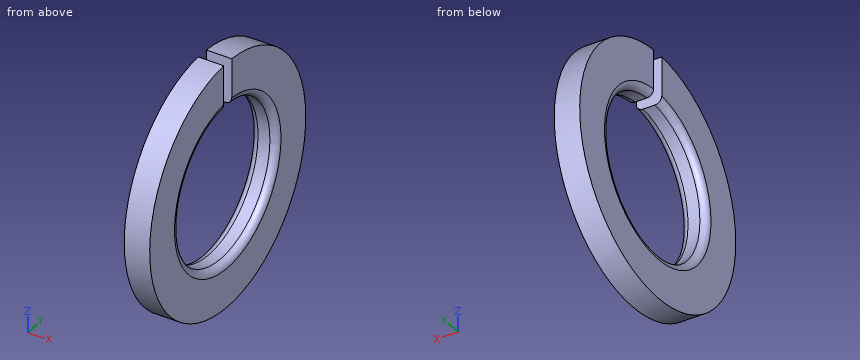
from build123d import *

# Parameters (mm, degrees)
SKETCH2_W = 3
SKETCH2_H = 29.682
GAP_DEPTH = 42.588700388


with BuildPart() as part:
    # Sketch1 → Base-Revolve (revolve)
    with BuildSketch(Plane.XY, mode=Mode.PRIVATE) as base_revolve_sk:
        with BuildLine():
            Line((0, 19.85), (0, 29.1))
            Line((0, 29.1), (-6, 29.1))
            Line((-6, 29.1), (-6, 19.85))
            ThreePointArc((-6, 19.85), (-5.53137085, 18.71862915), (-4.4, 18.25))
            Line((-4.4, 18.25), (-1.6, 18.25))
            ThreePointArc((-1.6, 18.25), (-0.46862915, 18.71862915), (0, 19.85))
        make_face()
    revolve(base_revolve_sk.sketch.rotate(Axis((-34.925, 0, 0), (1, 0, 0)), 90), axis=Axis((-34.925, 0, 0), (1, 0, 0)))

    # Sketch2 → Gap (cut, through all)
    with BuildSketch(Plane(origin=(0, 0, 0), x_dir=(0, -1, 0), z_dir=(-1, 0, 0))):
        with Locations((0, 14.841)):
            Rectangle(SKETCH2_W, SKETCH2_H)
    extrude(amount=GAP_DEPTH, mode=Mode.SUBTRACT)


solid = part.part
Here's how the part is built. I have some questions about the finished solid (model axes, mm). Round coordinates to 2 decimals unless told otherwise and drop trailing zeros. Loops run counter-clockwise (first coordinate to the right, second up) from the corner with the lowest first, then second, coordinate; pieces in that order, holes last. Notation, with made-up numbers: (83.25, -15.75) - (139.25, -15.75) arc R18 ccw to (139.25, 13.25) - close; hole circle Ø7 at (62.5, -20.5). An arc over 180 degrees is marked (long way). One line per question, with ' | ' between items. Start each with the question number.
Q1. I want a section at A-A (z = 0). Write out the boundary of the cut face in (x, y).
Q2. I want a section at B-B (y = 0). Write out the boundary of the cut face in (x, z).
Q3. Please list where these lines run through material, in increasing order: line 1 (Y direction, x = -2.25, z = 0); line 2 (Z direction, x = -2.5, y = -10); line 3 (Z direction, x = -3.75, y = -8.5). Write a range as [from, to].
Q4. I want a section at C-C (x = -3.5). Write out the boundary of the cut face in (y, z), then the cut area to 3 significant figures.
Q5. I want a section at D-D (z = 24). Write out the boundary of the cut face in (x, y), then the cut area to 3 significant figures.
Q6. Will these pins go through, and if not, where does the flat tip stop? pin 1 (1.5 mm diameter, centred on x = -3, z = -12, fed in from -Y); pin 2 (2 mm diameter, centred on x = -3.5, z = 23, fed in from -Y); pin 3 (1.8 mm diameter, centred on x = -3, z = 25.5, fed in from +Y).
Response values:
1) outline: (-6, -29.1) - (0, -29.1) - (0, -19.85) arc R1.6 ccw to (-1.6, -18.25) - (-4.4, -18.25) arc R1.6 ccw to (-6, -19.85) - close; (-6, 19.85) arc R1.6 ccw to (-4.4, 18.25) - (-1.6, 18.25) arc R1.6 ccw to (0, 19.85) - (0, 29.1) - (-6, 29.1) - close
2) outline: (-6, -29.1) - (0, -29.1) - (0, -19.85) arc R1.6 ccw to (-1.6, -18.25) - (-4.4, -18.25) arc R1.6 ccw to (-6, -19.85) - close
3) line 1: y = [-29.1, -18.25], [18.25, 29.1] | line 2: z = [-27.33, -15.27], [15.27, 27.33] | line 3: z = [-27.83, -16.15], [16.15, 27.83]
4) outline: (-1.5, 18.19) - (-1.5, 29.06) arc R29.1 ccw (long way) to (1.5, 29.06) - (1.5, 18.19) arc R18.25 cw (long way) to start | area: 1,580 mm²
5) outline: (-6, -16.46) - (0, -16.46) - (0, -1.5) - (-6, -1.5) - close; (-6, 1.5) - (0, 1.5) - (0, 16.46) - (-6, 16.46) - close | area: 179 mm²
6) pin 1: stops at y = -26.84 | pin 2: stops at y = -19.05 | pin 3: stops at y = 15.55
